Part print with two shaded views. Sizes in mm from the minimum x, y, z corner. A direction names the side the tool comes from. Give positions to 0.01 mm unless a question says otherwise; leave off trailing zeros. Order: outer loops, then holes, each group sorted by start corner. A loop starts at its lowest first (then second) coordinate and runs counter-clockwise, first axis right, second up. Notation, with made-up numbers: M 17.5,52.5 L 46.5,52.5 A27 cw 46.5,89.5 Z; hole C 15.5,72 d6. An arc over 180 degrees is marked long. Return JSON: item names as keys, results as strings.
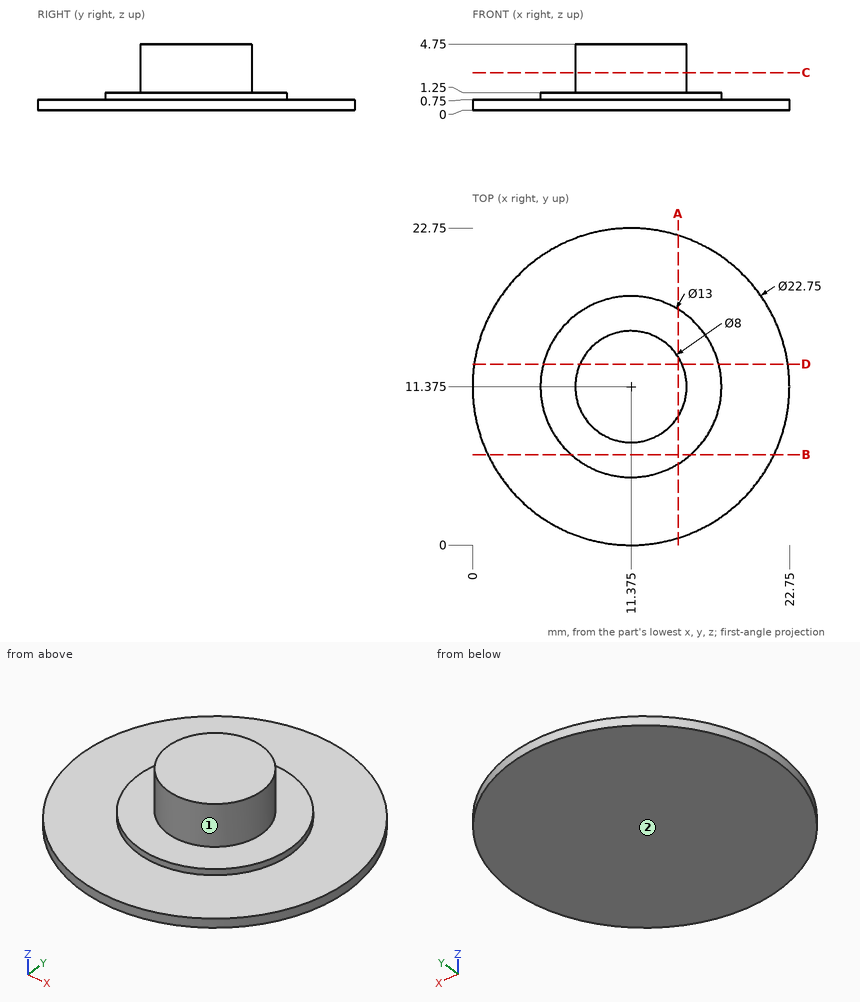
Q1. Band-saw the part on D-D (y = 13). Give the cut face in (x, z).
Established:
{"outline": "M 0.12,0 L 22.63,0 L 22.63,0.75 L 17.67,0.75 L 17.67,1.25 L 15.03,1.25 L 15.03,4.75 L 7.72,4.75 L 7.72,1.25 L 5.08,1.25 L 5.08,0.75 L 0.12,0.75 Z"}
Q2. Probe line 1 along Z through (x, y) = (16, 18.5); line 2 along Z through (x, y) = (14, 15.25); line 3 along Y through (x, z) = (11, 0.45). List the from-to ranges inside material, lowest first.
Established:
{"line 1": "z = 0 to 0.75", "line 2": "z = 0 to 1.25", "line 3": "y = 0.01 to 22.74"}
Q3. Band-saw the part on B-B (y = 6.5). Give the cut face in (x, z).
Established:
{"outline": "M 1.1,0 L 21.65,0 L 21.65,0.75 L 15.67,0.75 L 15.67,1.25 L 7.08,1.25 L 7.08,0.75 L 1.1,0.75 Z"}
Q4. Pin check, flat tips, straight feed: pin 1 (2 mm diameter, centred on y = 11.5, z = 4, fed in from -X) (3 decimals); pin 2 (1 mm diameter, centred on y = 13.5, z = 3, fed in from +X); pin 3 (1 mm diameter, centred on x = 18, z = 3.5, fed in from +Y); pin 4 (1 mm diameter, centred on x = 11.5, y = 4.5, fed in from +Z). Stop position of each tip, or through.
Established:
{"pin 1": "stops at x = 7.375", "pin 2": "stops at x = 15.03", "pin 3": "passes through", "pin 4": "stops at z = 1.25"}
Q5. Band-saw the part on C-C (z = 2.7). Give the cut face in (x, y) (3 decimals), then the cut area to 3 significant figures.
Established:
{"outline": "C 11.375,11.375 d8", "area": "50.3 mm²"}
Q6. 3-axis set-ups, long thin cutter, end or side, ignore diameter. For the marked faces 1 and 2: which of +Z, -Z, +X, -X, +Y, -Y reach the whole face in a straight line?
Established:
{"face 1": "+Z", "face 2": "-Z, +X, -X, +Y, -Y"}
Q7. Band-saw the part on A-A (x = 14.75). Give the cut face in (y, z).
Established:
{"outline": "M 0.51,0 L 22.24,0 L 22.24,0.75 L 16.93,0.75 L 16.93,1.25 L 13.52,1.25 L 13.52,4.75 L 9.23,4.75 L 9.23,1.25 L 5.82,1.25 L 5.82,0.75 L 0.51,0.75 Z"}
